Source: CAD feature listing. Evaluate the final solid. Frame: model axes, mm. Round coordinates to 2 decimals unless told otherwise and drop trailing zeros. Loops run counter-clockwise (first coordinate to the right, second up) from the corner with the lowest first, then second, coordinate; pieces in that order, holes last.
Item 1: Pull-direction query (Y, two-part tool) for faces 1 (the flat face through (-64, 31.75, 3)), 2 (the conical face through (-34.8, 8.1, 3.9)), 3 (the flat face through (-64, 13, 0)), 4 (the conical face through (-34.8, 24, 3.9)); classes: released by +Y, released by -Y, zero draft, split by the parting line, or undercut.
Item 2: Section query A-A on x = -63.5. Return loops of the section in (y, z) (3 decimals), then the cut area to 3 significant figures.
Item 3: First-contact query: P1, Ø9, axis at x = -88.69, y = 23.81, coming from the +Z side. Flat tip, straight axial feed; report the tip coordinate or a pass-through.
Item 4: Ray query, L1, parallel to Y at x = -63.5, z = 3.25 (3 decimals); L2, parallel to X at y = 9.5, z = 4.75; L3, parallel to Y at x = -36, z = 2.25. Return the intervals inside material, ascending.
Item 5: Section query B-B on z = 1.25. Give the number of separate pieces and of enclosed holes in the cut face, then the cut area to 3 significant figures.
```python
from build123d import *

# Parameters (mm, degrees)
SKETCH1_W                                           = 79.746162722
SKETCH1_H                                           = 31.75
SKETCH1_R                                           = 6.35
BOSS_EXTRUDE1_DEPTH                                 = 6.35
CSK_FOR_1_4_FLAT_HEAD_MACHINE_SCREW_100_D           = 6.7564
CSK_FOR_1_4_FLAT_HEAD_MACHINE_SCREW_100_CSINK_D     = 12.8778
CSK_FOR_1_4_FLAT_HEAD_MACHINE_SCREW_100_CSINK_ANGLE = 100


with BuildPart() as part:
    # Sketch1 → Boss-Extrude1 (new body)
    with BuildSketch(Plane.XY):
        with Locations((-63.5, 15.875)):
            Rectangle(SKETCH1_W, SKETCH1_H)
        with Locations((-63.5, 22.225)):
            Circle(SKETCH1_R, mode=Mode.SUBTRACT)
    extrude(amount=BOSS_EXTRUDE1_DEPTH)

    # CSK for 1/4 Flat Head Machine Screw (100)1 (through all)
    with Locations(Plane.XY.offset(6.35)):
        with Locations((-88.685760173, 23.8125), (-88.685760173, 7.9375), (-38.314239827, 7.9375), (-38.314239827, 23.8125)):
            CounterSinkHole(CSK_FOR_1_4_FLAT_HEAD_MACHINE_SCREW_100_D / 2, CSK_FOR_1_4_FLAT_HEAD_MACHINE_SCREW_100_CSINK_D / 2, counter_sink_angle=CSK_FOR_1_4_FLAT_HEAD_MACHINE_SCREW_100_CSINK_ANGLE)


solid = part.part
```
Data:
1. face 1: released by +Y
1. face 2: undercut
1. face 3: zero draft
1. face 4: undercut
2. outline: (0, 0) - (15.875, 0) - (15.875, 6.35) - (0, 6.35) - close; (28.575, 0) - (31.75, 0) - (31.75, 6.35) - (28.575, 6.35) - close
2. area: 121 mm2
3. P1: stops at z = 4.73
4. L1: y = 0 to 15.875, 28.575 to 31.75
4. L2: x = -103.37 to -92.94, -84.43 to -42.57, -34.06 to -23.63
4. L3: y = 0 to 5.48, 10.4 to 21.35, 26.27 to 31.75
5. separate pieces: 1
5. enclosed holes: 5
5. area: 2,260 mm2
